For this review, take the finished solid that the model builds, in its own axes (mm). A direction names the side the tool comes from. Round coordinates to 2 decimals unless told otherwise and drop trailing zeros. Order: outer loops, then holes, each group sorted by start corner. A loop starts at its lowest first (then second) coordinate and runs counter-clockwise, first axis right, second up. Notation, with made-up numbers: (68.25, -33.5) -> (105.25, -33.5) arc R16 ccw to (105.25, -18.5) -> close; hole circle Ø11 at (9.5, 64.5). An arc over 180 degrees is marked (long way). Use a Markdown table: item, result. Add a question column.
1) Draft analysis for pull direction Z (two halves, no side actions). For faces 5 (the face through (-16, 4, 3.95)), 6 (the face through (-7.15, 0.84, 0.62)), 7 (the face through (0, 0, 0)), state which applies: pulls with the +Z half, pulls with the -Z half, needs draft (parallel to the pull), parting line crosses it, or undercut.
2) Consider section D-D (z = 4.75). State the section outline as (x, y) points.
3) Consider section C-C (y = 2.25). State the section outline as (x, z) points.
4) Clearance check with flat-ended pins moving along their axes: P1, Ø1, axis at x = -1, y = 6.5, coming from the +Z side; P2, Ø8.5, axis at x = -18.5, z = -1.5, coming from the +Y side; P3, Ø0.8, axis at y = 0.5, z = -3.5, coming from the -X side. State where each tip first meets the part, or that it passes through.
5) Machinability: for faces 1 (the face through (5, 5, -6.4)), 2 (the face through (-16.1, 1, 0)), 3 (the face through (-16, 4, -3.95)), 4 (the face through (5, 5, 6.4)), which of the approach directions +Z, -Z, +X, -X, +Y, -Y give a long, thin tool a straight path to every point of the face, cutting with its end or side? Answer none if there is none.
6) Consider section A-A (z = 0). State the section outline as (x, y) points.
7) Consider section B-B (x = -5.95). State the section outline as (y, z) points, plus the area to 4 significant figures.
8) Wall thickness on line 1 along X through (y, z) = (2.5, 1.5); line 2 along X through (y, z) = (0.65, 0); line 3 along X through (y, z) = (2.5, 4.5): over which ranges is each line inside the solid? List them lowest first. Write a range as [from, to].
```python
from build123d import *

# Parameters (mm, degrees)
SKETCH1_W           = 32.2
SKETCH1_H           = 14.2
SKETCH1_R           = 1.35
BOSS_EXTRUDE1_DEPTH = 1.7
SKETCH2_W           = 16
SKETCH2_H           = 12.8
BOSS_EXTRUDE2_DEPTH = 6
SKETCH3_W           = 10.4
SKETCH3_H           = 7.9
BOSS_EXTRUDE3_DEPTH = 4.8


with BuildPart() as part:
    # Sketch1 → Boss-Extrude1 (new body)
    with BuildSketch(Plane(origin=(0, 0, 0), x_dir=(1, 0, 0), z_dir=(0, 1, 0))):
        Rectangle(SKETCH1_W, SKETCH1_H)
        with Locations(Location((-5.95, 0, 0), (0, 0, 270))):
            Circle(SKETCH1_R, mode=Mode.SUBTRACT)
    extrude(amount=BOSS_EXTRUDE1_DEPTH)

    # Sketch2 → Boss-Extrude2 (add)
    with BuildSketch(Plane(origin=(0, 1.7, 0), x_dir=(1, 0, 0), z_dir=(0, 1, 0))):
        with Locations((5, 0)):
            Rectangle(SKETCH2_W, SKETCH2_H)
    extrude(amount=BOSS_EXTRUDE2_DEPTH)

    # Sketch3 → Boss-Extrude3 (add)
    with BuildSketch(Plane(origin=(0, 1.7, 0), x_dir=(1, 0, 0), z_dir=(0, 1, 0))):
        with Locations((-16.1, 0)):
            Rectangle(SKETCH3_W, SKETCH3_H)
    extrude(amount=BOSS_EXTRUDE3_DEPTH)


solid = part.part
```
Results list:
| question | item | result |
|---|---|---|
| 1 | face 5 | pulls with the +Z half |
| 1 | face 6 | undercut |
| 1 | face 7 | needs draft |
| 2 | outline | (-16.1, 0) -> (16.1, 0) -> (16.1, 1.7) -> (13, 1.7) -> (13, 7.7) -> (-3, 7.7) -> (-3, 1.7) -> (-16.1, 1.7) -> close |
| 3 | outline | (-21.3, -3.95) -> (-10.9, -3.95) -> (-10.9, 3.95) -> (-21.3, 3.95) -> close; (-3, -6.4) -> (13, -6.4) -> (13, 6.4) -> (-3, 6.4) -> close |
| 4 | P1 | z = 6.4 |
| 4 | P2 | y = 6.5 |
| 4 | P3 | x = -16.1 |
| 5 | face 1 | -Z, +X, -X, +Y |
| 5 | face 2 | +Z, -Z, -X, -Y |
| 5 | face 3 | -Z, -X, +Y |
| 5 | face 4 | +Z, +X, -X, +Y |
| 6 | outline | (-21.3, 1.7) -> (-16.1, 1.7) -> (-16.1, 0) -> (-7.3, 0) -> (-7.3, 1.7) -> (-10.9, 1.7) -> (-10.9, 6.5) -> (-21.3, 6.5) -> close; (-4.6, 0) -> (16.1, 0) -> (16.1, 1.7) -> (13, 1.7) -> (13, 7.7) -> (-3, 7.7) -> (-3, 1.7) -> (-4.6, 1.7) -> close |
| 7 | outline | (0, -7.1) -> (1.7, -7.1) -> (1.7, -1.35) -> (0, -1.35) -> close; (0, 1.35) -> (1.7, 1.35) -> (1.7, 7.1) -> (0, 7.1) -> close |
| 7 | area | 19.55 mm2 |
| 8 | line 1 | [-21.3, -10.9], [-3, 13] |
| 8 | line 2 | [-16.1, -7.3], [-4.6, 16.1] |
| 8 | line 3 | [-3, 13] |
